from build123d import *

# Parameters (mm, degrees)
BOSS_EXTRUDE1_DEPTH   = 1
BOSS_EXTRUDE2_DEPTH   = 6
SKETCH4_R             = 1.5
SKETCH4_W             = 6.5
SKETCH4_H             = 6.5
SKETCH4_W_2           = 3.913005348
SKETCH4_H_2           = 6.097566615
BOSS_EXTRUDE6_DEPTH   = 1
FILLET1_R             = 0.25
BOSS_EXTRUDE7_DEPTH   = 3.5
SKETCH6_R             = 6.25
BOSS_EXTRUDE8_DEPTH   = 4
SKETCH7_R             = 0.5
BOSS_EXTRUDE9_DEPTH   = 1
CHAMFER1_SIZE         = 0.75
CHAMFER1_SIZE2        = 0.349730744
CHAMFER1_PART_2_SIZE  = 0.75
CHAMFER1_PART_2_SIZE2 = 0.349730744


with BuildPart() as part:
    # Sketch1 → Boss-Extrude1 (new body)
    with BuildSketch(Plane(origin=(0, 0, 0), x_dir=(1, 0, 0), z_dir=(0, 1, 0))):
        with BuildLine():
            Line((-3.354101966, 11), (3.354101966, 11))
            ThreePointArc((3.354101966, 11), (7.611619318, 8.620513404), (10.5, 4.69041576))
            Line((10.5, 4.69041576), (10.5, -4.69041576))
            ThreePointArc((10.5, -4.69041576), (7.611619318, -8.620513404), (3.354101966, -11))
            Line((3.354101966, -11), (-3.354101966, -11))
            ThreePointArc((-3.354101966, -11), (-7.611619318, -8.620513404), (-10.5, -4.69041576))
            Line((-10.5, -4.69041576), (-10.5, 4.69041576))
            ThreePointArc((-10.5, 4.69041576), (-7.611619318, 8.620513404), (-3.354101966, 11))
        make_face()
    extrude(amount=BOSS_EXTRUDE1_DEPTH)

    # Sketch2 → Boss-Extrude2 (add)
    with BuildSketch(Plane.XZ):
        Polygon((8.109719748, -2.570195786), (10.184176938, -4.737366146), (4.405055978, -10.269251985), (2.330598788, -8.102081625), align=None)
    extrude(amount=BOSS_EXTRUDE2_DEPTH)

    # Sketch4 → Boss-Extrude6 (add)
    with BuildSketch(Plane.XZ):
        with Locations((0, -9)):
            Circle(SKETCH4_R)
        with Locations((0, 9)):
            Circle(SKETCH4_R)
        with Locations((1.885591241, -1.931388967)):
            Rectangle(SKETCH4_W, SKETCH4_H)
        Polygon((-6.789671936, 7.633587439), (-2.564617425, 4.781139469), (-5.233344576, 0.828212788), (-9.458399087, 3.680660758), align=None)
        with Locations((-6.013545028, -4.933267479)):
            Rectangle(SKETCH4_W_2, SKETCH4_H_2)
        with BuildLine():
            Line((7.537936682, 4.261094781), (8.522189561, 4.261094781))
            ThreePointArc((8.522189561, 4.261094781), (8.906288246, 3.876996096), (8.522189561, 3.492897412))
            Line((8.522189561, 3.492897412), (7.537936682, 3.492897412))
            ThreePointArc((7.537936682, 3.492897412), (7.153837998, 3.876996096), (7.537936682, 4.261094781))
        make_face()
        with BuildLine():
            Line((7.549939766, 3.276841902), (8.534192645, 3.276841902))
            ThreePointArc((8.534192645, 3.276841902), (8.918291329, 2.892743217), (8.534192645, 2.508644533))
            Line((8.534192645, 2.508644533), (7.549939766, 2.508644533))
            ThreePointArc((7.549939766, 2.508644533), (7.165841082, 2.892743217), (7.549939766, 3.276841902))
        make_face()
        with BuildLine():
            Line((7.393899676, 0.228058594), (8.378152554, 0.228058594))
            ThreePointArc((8.378152554, 0.228058594), (8.762251239, -0.156040091), (8.378152554, -0.540138775))
            Line((8.378152554, -0.540138775), (7.393899676, -0.540138775))
            ThreePointArc((7.393899676, -0.540138775), (7.009800991, -0.156040091), (7.393899676, 0.228058594))
        make_face()
        with BuildLine():
            Line((7.405902759, -0.756194285), (8.390155638, -0.756194285))
            ThreePointArc((8.390155638, -0.756194285), (8.774254323, -1.140292969), (8.390155638, -1.524391654))
            Line((8.390155638, -1.524391654), (7.405902759, -1.524391654))
            ThreePointArc((7.405902759, -1.524391654), (7.021804075, -1.140292969), (7.405902759, -0.756194285))
        make_face()
    extrude(amount=BOSS_EXTRUDE6_DEPTH)

    # Fillet1
    fillet1_edges = [part.edges().sort_by_distance(p)[0] for p in [
        (-1.5, -1, -9),
        (-1.5, -1, 9),
    ]]
    fillet(fillet1_edges, radius=FILLET1_R)

    # Sketch5 → Boss-Extrude7 (add)
    with BuildSketch(Plane(origin=(0, 1, 0), x_dir=(1, 0, 0), z_dir=(0, 1, 0))):
        with BuildLine():
            Line((-2, -6.25), (-2, -9))
            ThreePointArc((-2, -9), (0, -11), (2, -9))
            Line((2, -9), (2, -6.25))
            Line((2, -6.25), (6.25, -6.25))
            Line((6.25, -6.25), (6.25, 6.25))
            Line((6.25, 6.25), (2, 6.25))
            Line((2, 6.25), (2, 9))
            ThreePointArc((2, 9), (0, 11), (-2, 9))
            Line((-2, 9), (-2, 6.25))
            Line((-2, 6.25), (-6.25, 6.25))
            Line((-6.25, 6.25), (-6.25, -6.25))
            Line((-6.25, -6.25), (-2, -6.25))
        make_face()
    extrude(amount=BOSS_EXTRUDE7_DEPTH)

    # Sketch6 → Boss-Extrude8 (add)
    with BuildSketch(Plane(origin=(0, 4.5, 0), x_dir=(1, 0, 0), z_dir=(0, 1, 0))):
        Circle(SKETCH6_R)
    extrude(amount=BOSS_EXTRUDE8_DEPTH)

    # Sketch7 → Boss-Extrude9 (add)
    with BuildSketch(Plane(origin=(0, 4.5, 0), x_dir=(1, 0, 0), z_dir=(0, 1, 0))):
        with Locations((0, 9)):
            Circle(SKETCH7_R)
        with Locations((0, -9)):
            Circle(SKETCH7_R)
    extrude(amount=BOSS_EXTRUDE9_DEPTH)

    # Chamfer1
    chamfer1_edges = [part.edges().sort_by_distance(p)[0] for p in [
        (-0.5, 5.5, -9),
    ]]
    chamfer1_side = [part.faces().sort_by_distance(p)[0] for p in [
        (-0.5, 5, -9),
    ]]
    chamfer(chamfer1_edges, length=CHAMFER1_SIZE, length2=CHAMFER1_SIZE2, reference=chamfer1_side[0])

    # Chamfer1 part 2
    chamfer1_part_2_edges = [part.edges().sort_by_distance(p)[0] for p in [
        (-0.5, 5.5, 9),
    ]]
    chamfer1_part_2_side = [part.faces().sort_by_distance(p)[0] for p in [
        (-0.5, 5, 9),
    ]]
    chamfer(chamfer1_part_2_edges, length=CHAMFER1_PART_2_SIZE, length2=CHAMFER1_PART_2_SIZE2, reference=chamfer1_part_2_side[0])

    # Sketch8 → Revolve1 (revolve)
    with BuildSketch(Plane.XY):
        with BuildLine():
            Line((0, 4.5), (0, 16.5))
            Line((0, 16.5), (0, 16.525))
            ThreePointArc((0, 16.525), (3.359575443, 16.092432155), (6.5, 14.822945763))
            Line((6.5, 14.822945763), (6.5, 14.797945763))
            ThreePointArc((6.5, 14.797945763), (7.136161739, 14.416457997), (7.75, 14))
            Line((7.75, 14), (7.75, 11.5))
            Line((7.75, 11.5), (5.75, 11.5))
            Line((5.75, 11.5), (5.75, 4.5))
            Line((5.75, 4.5), (0, 4.5))
        make_face()
    revolve(axis=Axis((0, 4.5, 0), (0, 1, 0)))


solid = part.part
The model under review builds one solid part; all positions refer to its coordinate system, in mm. A direction names the side the tool comes from. Give positions to 0.01 mm unless a question says otherwise; leave off trailing zeros. Order: outer loops, then holes, each group sorted by start corner. A loop starts at its lowest first (then second) coordinate and runs counter-clockwise, first axis right, second up. Notation, with made-up numbers: M 77,82.25 L 118,82.25 A11 ccw 118,98.25 Z; hole C 23,61.5 d1. An arc over 180 degrees is marked long. One line per question, with ' | ' between items. Start each with the question number.
1) Consider section A-A, the plane y = 12.25. Give the boundary of the cut face in (x, z).
2) Consider section B-B, the plane y = -2.25. Give the boundary of the cut face in (x, z), then the cut area to 3 significant figures.
3) For faces 5 (the face through (-7.316, -0.493, 2.234)), 6 (the face through (7.9, -0.5, -0.756)), 7 (the face through (-6, -0.5, -7.982)), list the 3-axis set-ups (+Z, -Z, +X, -X, +Y, -Y) from which the entire face can be reached by the end or side of a thin tool; tool diameter is ignored.
4) Clearance check with flat-ended pins moving along their axes: P1, Ø3, axis at x = -4.5, y = 2, coming from the +Z side; P2, Ø0.5, axis at x = 8, y = -0.5, coming from the -Z side; P3, Ø1.1, axis at y = -0.5, z = -3.5, coming from the +X side; P4, Ø1.2, axis at x = -0.5, z = 9.5, coming from the -Y side. State where each tip first meets the part, or that it passes through.
5) Wall thickness on L1, parallel to X at y = 2.5, z = 5.25; L2, parallel to Z at x = 0.25, y = 12.25; L3, parallel to Y at x = 8, z = -3.25: over which ranges is each line inside the solid? List them lowest first. Write a range as from..to.
6) Mouldability with a two-part tool opening along Z and no side actions: class faces 1 (the face through (-6, -1, 4)), 2 (the face through (-3.9, -0.5, 2.8)), 3 (the face through (8, -0.5, 3.277)), 4 (the face through (-7.56, 0.493, 8.666)) as pulls with the +Z half, pulls with the -Z half, needs draft (parallel to the pull), parting line crosses it, or undercut.
Found:
1) outline: C 0,0 d15.5
2) outline: M 2.33,-8.1 L 4.41,-10.27 L 10.18,-4.74 L 8.11,-2.57 Z | area: 24.0 mm²
3) face 5: -X, -Y | face 6: +X, -Y | face 7: -Z, -X, -Y
4) P1: stops at z = 10.99 | P2: stops at z = -7.07 | P3: stops at x = 10.5 | P4: stops at y = -1
5) L1: x = -6.25..6.25 | L2: z = -7.75..7.75 | L3: y = -6..1
6) face 1: needs draft | face 2: undercut | face 3: undercut | face 4: pulls with the +Z half
